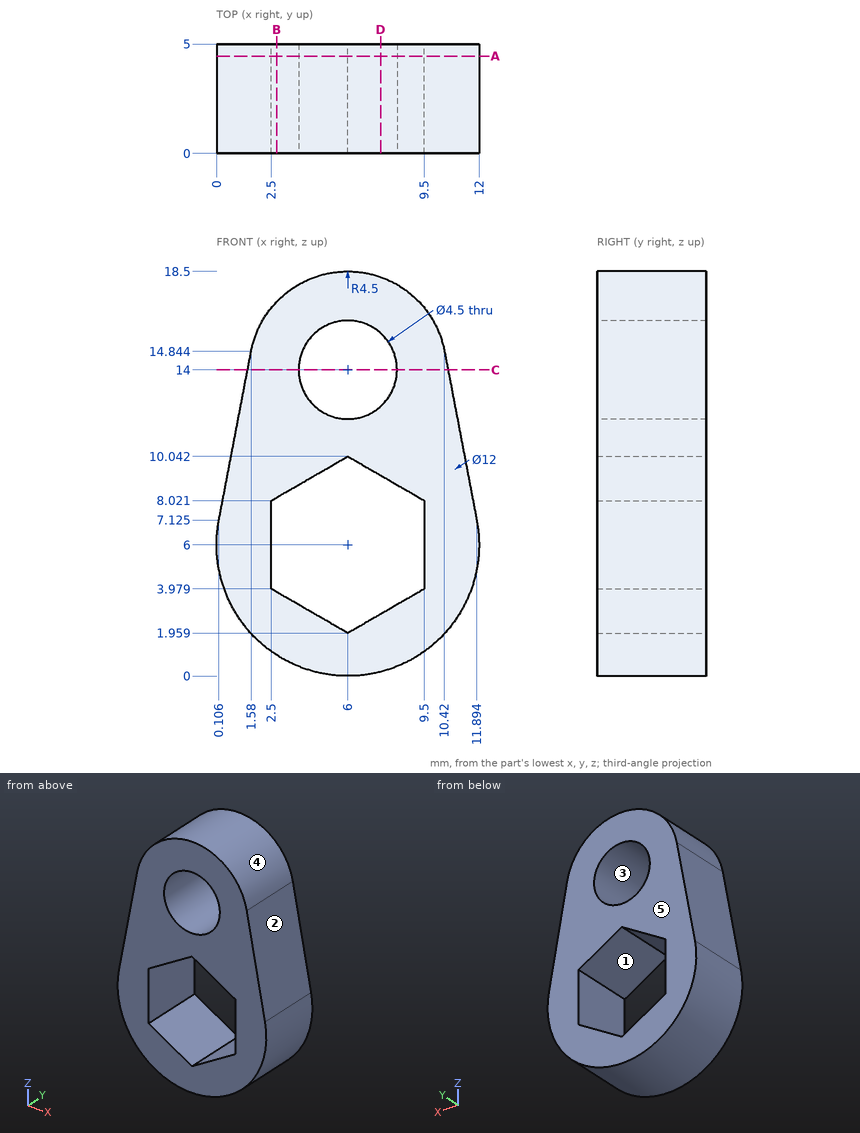
Part print with two shaded views. Sizes in mm from the minimum x, y, z corner. A direction names the side the tool comes from. Coordinates: 2 decimals unless noted, no trailing zeros. Loops run counter-clockwise (first coordinate to the right, second up) from the corner with the lowest first, then second, coordinate; pieces in that order, holes last. Notation, with made-up numbers: M 72,4.25 L 102,4.25 A11 ccw 102,9.25 Z; hole C 23,78.25 d9. An arc over 180 degrees is marked long. Use CSV: the item, a comma, the result in double quotes. Start each with the question number.
1. Band-saw the part on C-C, the plane z = 14. List the corners of the cut face in (x, y), then the cut area to 3 significant figures.
2. Band-saw the part on A-A, the plane y = 4.45. Give the number of separate pieces and of enclosed holes in the cut face.
3. Band-saw the part on B-B, the plane x = 2.75. List the corners of the cut face in (y, z) (1 decimal).
4. Two-plate mould, pull along Z, no slides. Class the marked faces 3, 4 and 5: pulls with the +Z half, pulls with the -Z half, needs draft (parallel to the pull), parting line crosses it, or undercut.
5. Tool access for the marked faces 1 and 2: list every direction of +Z, -Z, +X, -X, +Y, -Y with a clear straight run to the whole face (end or side of a thin tool).
6. Flat gauge pins, fed straight in: pin 1 (1 mm diameter, centred on y = 1, z = 4.5, fed in from -X); pin 2 (3 mm diameter, centred on x = 1.5, z = 15.5, fed in from -Y); pin 3 (1 mm diameter, centred on x = 10.5, y = 4, fed in from +Z). Where does each tip first touch, or does it go through?
7. Probe probe 1 along Z at (x, y) = (5.5, 3.1) (1 decimal); probe 2 along X at (y, z) = (2.5, 9.25) (1 decimal); probe 3 along Z at (x, y) = (8, 0.45) (1 decimal). List the from-to ranges inside material, lowest first. Write a range as [from, to].
8. Band-saw the part on D-D, the plane x = 7.5. List the corners of the cut face in (y, z) (1 decimal).
Entries:
1,outline,"M 1.42,0 L 3.75,0 L 3.75,5 L 1.42,5 Z; M 8.25,0 L 10.58,0 L 10.58,5 L 8.25,5 Z"
1,area,"23.3 mm2"
2,separate pieces,"1"
2,enclosed holes,"2"
3,outline,"M 0,1 L 5,1 L 5,3.8 L 0,3.8 Z; M 0,8.2 L 5,8.2 L 5,17.1 L 0,17.1 Z"
4,face 3,"undercut"
4,face 4,"pulls with the +Z half"
4,face 5,"needs draft"
5,face 1,"+Y, -Y"
5,face 2,"+Z, +X, +Y, -Y"
6,pin 1,"stops at x = 0.08"
6,pin 2,"stops at y = 0"
6,pin 3,"stops at z = 16.06"
7,probe 1,"z = [0, 2.2], [9.8, 11.8], [16.2, 18.5]"
7,probe 2,"x = [0.5, 4.6], [7.4, 11.5]"
7,probe 3,"z = [0.3, 3.1], [8.9, 13], [15, 18]"
8,outline,"M 0,0.2 L 5,0.2 L 5,2.8 L 0,2.8 Z; M 0,9.2 L 5,9.2 L 5,12.3 L 0,12.3 Z; M 0,15.7 L 5,15.7 L 5,18.2 L 0,18.2 Z"
